Print and shaded views of the part. All mm, measured from the part's lowest x, y and z. Coordinates: 2 decimals unless noted, no trailing zeros. Order: outer loops, then holes, each group sorted by start corner. A loop starts at its lowest first (then second) coordinate and runs counter-clockwise, first axis right, second up. Notation, with made-up numbers: (54, 24) -> (59, 24) arc R20 ccw to (59, 55) -> close; hole circle Ø9 at (-18.75, 78.25). An arc over 180 degrees is marked (long way). Return JSON: item names as keys, results as strings. Group by question number.
1) Probe line 1 (Y direction, x = 19.05, z = 1.25); line 2 (X direction, y = 57.15, z = 1.05); line 3 (Y direction, x = 18.5, z = 3.5) (1 decimal). List the from-to ranges inside material, lowest first.
2) Cut at A-A (y = 57.15). Write the cut outline in (x, z), and give its area (3 significant figures).
3) Cut at B-B (x = 19.05). Write the cut outline in (y, z), and give its area (3 significant figures).
4) Cut at D-D (y = 19.05). Write the cut outline in (x, z).
5) Flat gauge pins, fed straight in: pin 1 (11 mm diameter, centred on x = 19.05, y = 57.15, fed in from +Z); pin 2 (5.5 mm diameter, centred on x = 19, y = 21, fed in from +Z). Where does each tip first touch, or does it go through?
6) Cut at C-C (z = 1.75). Write the cut outline in (x, y), and give its area (3 significant figures).
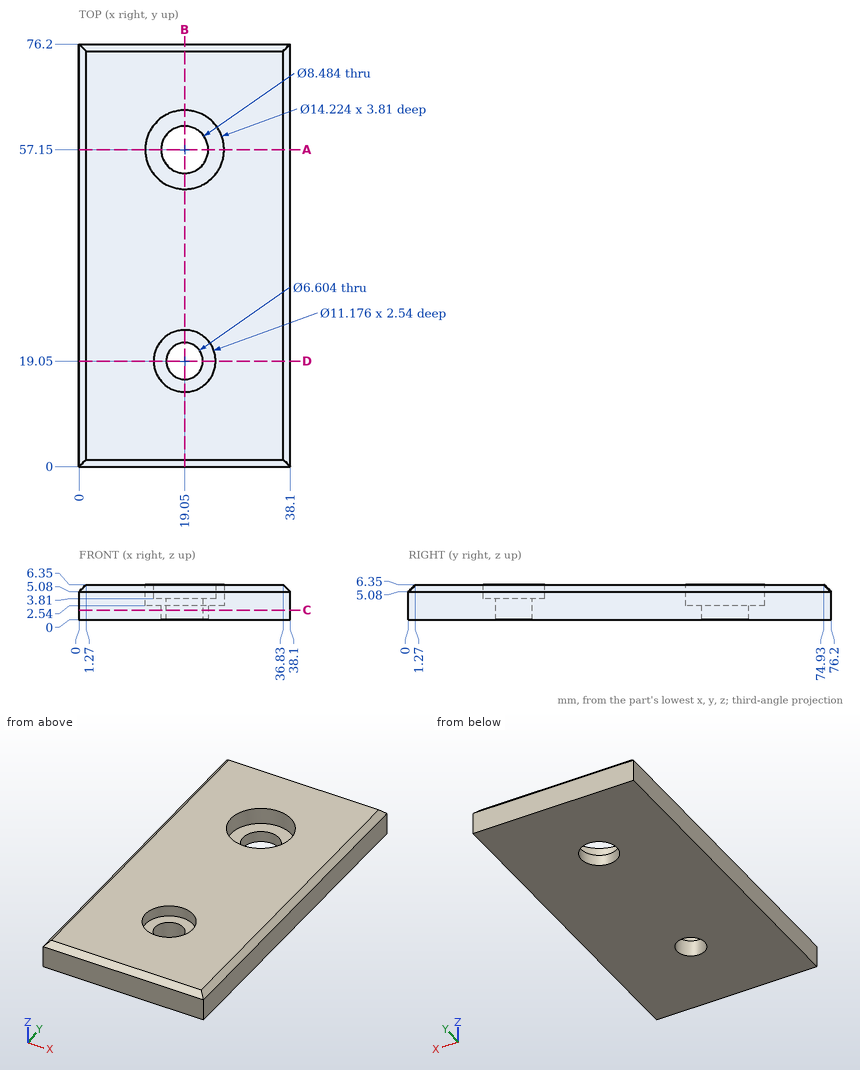
Answers below:
{
 "1": {"line 1": "y = 0 to 15.75, 22.35 to 52.91, 61.39 to 76.2", "line 2": "x = 0 to 14.81, 23.29 to 38.1", "line 3": "y = 0 to 15.8, 22.3 to 50.1, 64.2 to 76.2"},
 "2": {"outline": "(0, 0) -> (14.81, 0) -> (14.81, 2.54) -> (11.94, 2.54) -> (11.94, 6.35) -> (1.27, 6.35) -> (0, 5.08) -> close; (23.29, 0) -> (38.1, 0) -> (38.1, 5.08) -> (36.83, 6.35) -> (26.16, 6.35) -> (26.16, 2.54) -> (23.29, 2.54) -> close", "area": "165 mm^2"},
 "3": {"outline": "(0, 0) -> (15.75, 0) -> (15.75, 3.81) -> (13.46, 3.81) -> (13.46, 6.35) -> (1.27, 6.35) -> (0, 5.08) -> close; (22.35, 0) -> (52.91, 0) -> (52.91, 2.54) -> (50.04, 2.54) -> (50.04, 6.35) -> (24.64, 6.35) -> (24.64, 3.81) -> (22.35, 3.81) -> close; (61.39, 0) -> (76.2, 0) -> (76.2, 5.08) -> (74.93, 6.35) -> (64.26, 6.35) -> (64.26, 2.54) -> (61.39, 2.54) -> close", "area": "353 mm^2"},
 "4": {"outline": "(0, 0) -> (15.75, 0) -> (15.75, 3.81) -> (13.46, 3.81) -> (13.46, 6.35) -> (1.27, 6.35) -> (0, 5.08) -> close; (22.35, 0) -> (38.1, 0) -> (38.1, 5.08) -> (36.83, 6.35) -> (24.64, 6.35) -> (24.64, 3.81) -> (22.35, 3.81) -> close"},
 "5": {"pin 1": "stops at z = 2.54", "pin 2": "stops at z = 3.81"},
 "6": {"outline": "(0, 0) -> (38.1, 0) -> (38.1, 76.2) -> (0, 76.2) -> close; hole circle Ø8.48 at (19.05, 57.15); hole circle Ø6.6 at (19.05, 19.05)", "area": "2,810 mm^2"}
}
